Build history of the part. All positions in model axes, mm. A direction names the side the tool comes from. Coordinates: 2 decimals unless noted, no trailing zeros. Loops run counter-clockwise (first coordinate to the right, second up) from the corner with the lowest first, then second, coordinate; pieces in that order, holes last.
(1) Slice it at D-D (y = 2.5). Give the cut face in (x, z), and give its area (3 significant figures).
(2) Tool access for faces 1 (the face through (-22, 8, -1)), 2 (the face through (-22, 0, -1)), 3 (the face through (-40, -3, -1)): list every direction of +Z, -Z, +X, -X, +Y, -Y with a clear straight run to the whole face (end or side of a thin tool).
(3) Slice it at C-C (y = 7). Give the cut face in (x, z), and give its area (3 significant figures).
(4) Slice it at A-A (x = -37.75). Give the cut face in (y, z).
(5) Flat gauge pins, fed straight in: P1, Ø0.5, axis at y = -3.5, z = -1, coming from the +X side; P2, Ø0.7, axis at x = -21, z = -0.5, coming from the -Y side. Where does each tip first touch, or does it go through?
(6) Slice it at B-B (z = -0.8). Give the cut face in (x, y), and give its area (3 significant figures).
(7) Wall check: L1, parallel to Y at x = -36.25, z = -0.9; L2, parallel to X at y = -3.25, z = -0.6; L3, parallel to X at y = 6.75, z = -1.2. Give the ranges that are in metal, low to high.
(8) Two-plate mould, pull along Y, no slides. Class faces 4 (the face through (-44.5, -1, -1)), 5 (the face through (-21, 5.864, -1)), 6 (the face through (-20.2, 5, -1)): pulls with the +Y half, pulls with the -Y half, needs draft (parallel to the pull), parting line crosses it, or undercut.
from build123d import *

# Parameters (mm, degrees)
SKETCH1_R           = 50
BOSS_EXTRUDE1_DEPTH = 2
SKETCH1_3_W         = 9
SKETCH1_3_H         = 4
BOSS_EXTRUDE2_DEPTH = 5
CUT_EXTRUDE1_DEPTH  = 9
SKETCH5_W           = 24
SKETCH5_H           = 2
BOSS_EXTRUDE3_DEPTH = 2.5
CUT_EXTRUDE7_DEPTH  = 2
SKETCH8_W           = 33
SKETCH8_H           = 2
BOSS_EXTRUDE4_DEPTH = 2.5
SKETCH13_W          = 24
SKETCH13_H          = 2.5
CUT_EXTRUDE10_DEPTH = 4
SKETCH1_9_R         = 10
CUT_EXTRUDE17_DEPTH = 2
CHAMFER2_SIZE       = 4.5
CHAMFER2_SIZE_2     = 3.150933922
CUT_EXTRUDE19_DEPTH = 9
SKETCH15_W          = 9
SKETCH15_H          = 3
SKETCH15_H_2        = 1
CUT_EXTRUDE20_DEPTH = 2
BOSS_EXTRUDE6_DEPTH = 1.8
FILLET4_R           = 0.5


with BuildPart() as part:
    # Sketch1 → Boss-Extrude1 (new body)
    with BuildSketch(Plane.XY):
        Circle(SKETCH1_R)
    extrude(amount=-BOSS_EXTRUDE1_DEPTH)

    # Sketch1<3> → Boss-Extrude2 (add)
    with BuildSketch(Plane.XY):
        with Locations((-40, 0)):
            Rectangle(SKETCH1_3_W, SKETCH1_3_H)
    extrude(amount=BOSS_EXTRUDE2_DEPTH)

    # Sketch4 → Cut-Extrude1 (cut)
    with BuildSketch(Plane.ZY.offset(44.5)):
        Polygon((0, 0), (2.5, 0), (2.5, -2), (5, -2), (5, 2), (0, 2), align=None)
        Polygon((0, 0), (0, -2), (2.5, 0), align=None)
    extrude(amount=-CUT_EXTRUDE1_DEPTH, mode=Mode.SUBTRACT)


with BuildPart() as cut_extrude1_piece_1:
    # of the separate pieces the step leaves, piece 1, a body of its own (cut_extrude1_pieces)
    add(part.part.solids().sort_by_distance((50, 0, 0))[0])

    # Sketch5 → Boss-Extrude3 (add)
    with BuildSketch(Plane.XY):
        with Locations((-23.5, -1)):
            Rectangle(SKETCH5_W, SKETCH5_H)
    extrude(amount=BOSS_EXTRUDE3_DEPTH)

    # Sketch1<4> → Cut-Extrude7 (cut)
    with BuildSketch(Plane.XY):
        with BuildLine():
            Line((10, 0), (0, 0))
            Line((0, 0), (-10, 0))
            ThreePointArc((-10, 0), (0, -10), (10, 0))
        make_face()
        with BuildLine():
            Line((-10, 0), (0, 0))
            Line((0, 0), (10, 0))
            ThreePointArc((10, 0), (0, 10), (-10, 0))
        make_face()
        with BuildLine():
            Line((10, 0), (0, 0))
            Line((0, 0), (-10, 0))
            ThreePointArc((-10, 0), (0, -10), (10, 0))
        make_face()
        with BuildLine():
            Line((-10, 0), (0, 0))
            Line((0, 0), (10, 0))
            ThreePointArc((10, 0), (0, 10), (-10, 0))
        make_face()
    extrude(amount=-CUT_EXTRUDE7_DEPTH, mode=Mode.SUBTRACT)



with BuildPart() as cut_extrude1_piece_2:
    # of the separate pieces the step leaves, piece 2, a body of its own (cut_extrude1_pieces)
    add(part.part.solids().sort_by_distance((-44.5, -2, 2.5))[0])


with BuildPart() as cut_extrude1_piece_1_1:
    add(cut_extrude1_piece_1.part)

    add(cut_extrude1_piece_2.part)  # Boss-Extrude4 merges Cut-Extrude1 piece 2
    # Sketch8 → Boss-Extrude4 (add)
    with BuildSketch(Plane.XY):
        with Locations((-28, -3)):
            Rectangle(SKETCH8_W, SKETCH8_H)
    extrude(amount=BOSS_EXTRUDE4_DEPTH)

    # Sketch13 → Cut-Extrude10 (cut)
    with BuildSketch(Plane(origin=(0, 0, 0), x_dir=(1, 0, 0), z_dir=(0, 1, 0))):
        with Locations((-23.5, -1.25)):
            Rectangle(SKETCH13_W, SKETCH13_H)
    extrude(amount=-CUT_EXTRUDE10_DEPTH, mode=Mode.SUBTRACT)

    # Sketch1<9> → Cut-Extrude17 (cut)
    with BuildSketch(Plane.XY):
        with BuildLine():
            Line((-22, 9.9), (-22, -9.9))
            Line((-22, -9.9), (-49.010101, -9.9))
            ThreePointArc((-49.010101, -9.9), (50, 0), (-49.010101, 9.9))
            Line((-49.010101, 9.9), (-22, 9.9))
        make_face()
        Circle(SKETCH1_9_R, mode=Mode.SUBTRACT)
    extrude(amount=-CUT_EXTRUDE17_DEPTH, mode=Mode.SUBTRACT)

    # Chamfer2
    # the kernel refuses this chamfer: 4.5, 3.150933922 mm, written as the material it takes off along each edge
    with BuildSketch(Plane(origin=(-35.5, -9.259884147, -9.074855184), x_dir=(-0.9997533347641299, 0.017342841849466925, -0.013874273479573545), z_dir=(0, 0.6246950475544244, 0.7808688094430303))) as chamfer2_piece_1_section:
        Polygon((CHAMFER2_SIZE * 0.999753334764, CHAMFER2_SIZE * 0.0222096741985), (-CHAMFER2_SIZE_2 * 0.0222096741981, CHAMFER2_SIZE_2 * 0.999753334746), (0, 0), align=None)
    chamfer2_piece_1 = extrude(amount=26.444532191, mode=Mode.PRIVATE)
    chamfer2_piece_1 = split(chamfer2_piece_1, bisect_by=Plane(origin=(-37.088065075, -2.140732647, 0), z_dir=(0, 0, 1)), keep=Keep.TOP, mode=Mode.PRIVATE)
    add(chamfer2_piece_1, mode=Mode.SUBTRACT)

    # Sketch17 → Cut-Extrude19 (cut)
    with BuildSketch(Plane.ZY.offset(44.5)):
        Polygon((0, -4), (2.5, -4), (2.5, 0), (0, -2), align=None)
    extrude(amount=-CUT_EXTRUDE19_DEPTH, mode=Mode.SUBTRACT)

    # Sketch15 → Cut-Extrude20 (cut)
    with BuildSketch(Plane(origin=(0, 0, -2), x_dir=(-1, 0, 0), z_dir=(0, 0, -1))):
        with Locations((40, -0.5)):
            Rectangle(SKETCH15_W, SKETCH15_H)
        with Locations((40, -3.5)):
            Rectangle(SKETCH15_W, SKETCH15_H_2)
    extrude(amount=-CUT_EXTRUDE20_DEPTH, mode=Mode.SUBTRACT)

    # Sketch18 → Boss-Extrude6 (add)
    with BuildSketch(Plane(origin=(-22, 0, 0), x_dir=(0, 0, -1), z_dir=(1, 0, 0))):
        Polygon((0, 4.064201772), (2, 4.064201772), (2, 5.864201772), (1, 5.864201772), (0, 5.864201772), align=None)
        Polygon((2, -5.869107155), (2, -4.069107155), (0, -4.069107155), (0, -5.869107155), (1, -5.869107155), align=None)
    extrude(amount=BOSS_EXTRUDE6_DEPTH)

    # Fillet4
    fillet4_edges = [cut_extrude1_piece_1_1.edges().sort_by_distance(p)[0] for p in [
        (-44.5, -0.5, 0),
        (-35.5, -0.5, 0),
        (-40, 1, 0),
        (-20.2, 5.864201772, -1),
        (-20.2, 4.064201772, -1),
        (-20.2, -4.069107155, -1),
        (-20.2, -5.869107155, -1),
        (-22, -9.9, -1),
        (-22, 9.9, -1),
    ]]
    fillet(fillet4_edges, radius=FILLET4_R)


solid = cut_extrude1_piece_1_1.part
Response values:
1. outline: (-49.94, -2) - (-22, -2) - (-22, 0) - (-49.94, 0) - close
1. area: 55.9 mm2
2. face 1: +Z, -Z, +X, +Y
2. face 2: +Z, -Z, +X
2. face 3: +Z, -Z
3. outline: (-49.51, -2) - (-22, -2) - (-22, 0) - (-49.51, 0) - close
3. area: 55.0 mm2
4. outline: (-9.9, -2) - (-4, -2) - (-4, 0) - (-9.9, 0) - close; (-3, -2) - (-2, -2) - (-2, 0) - (-3, 0) - close; (1, -2) - (9.9, -2) - (9.9, 0) - (1.5, 0) arc R0.5 ccw to (1, -0.5) - close
5. P1: stops at x = -22
5. P2: stops at y = -5.87
6. outline: (-49.01, -9.9) - (-22.5, -9.9) arc R0.5 ccw to (-22, -9.4) - (-22, -5.87) - (-20.7, -5.87) arc R0.5 ccw to (-20.2, -5.37) - (-20.2, -4.57) arc R0.5 ccw to (-20.7, -4.07) - (-22, -4.07) - (-22, 4.06) - (-20.7, 4.06) arc R0.5 ccw to (-20.2, 4.56) - (-20.2, 5.36) arc R0.5 ccw to (-20.7, 5.86) - (-22, 5.86) - (-22, 9.4) arc R0.5 ccw to (-22.5, 9.9) - (-49.01, 9.9) arc R50 ccw to start; hole (-44.5, -4) - (-35.5, -4) - (-35.5, -3) - (-44.5, -3) - close; hole (-44.5, -2) - (-35.5, -2) - (-35.5, 1) - (-44.5, 1) - close
6. area: 518 mm2
7. L1: y = -9.9 to -4, -3 to -2, 1 to 9.9
7. L2: x = -49.89 to -44.5, -35.5 to -22
7. L3: x = -49.54 to -22
8. face 4: undercut
8. face 5: pulls with the +Y half
8. face 6: needs draft
